Work out the finished part from the listing and answer in its coordinate system (mm). Round coordinates to 2 decimals unless told otherwise and drop trailing zeros. Order: outer loops, then holes, each group sorted by start corner. A loop starts at its lowest first (then second) coordinate and runs counter-clockwise, first axis right, second up. Notation, with made-up numbers: (-28.5, 76.25) - (12.5, 76.25) arc R17 cw to (12.5, 81.25) - close; hole circle Ø8 at (-33, -39.5). An arc over 180 degrees is marked (long way). Put each result on its own line as item: value.
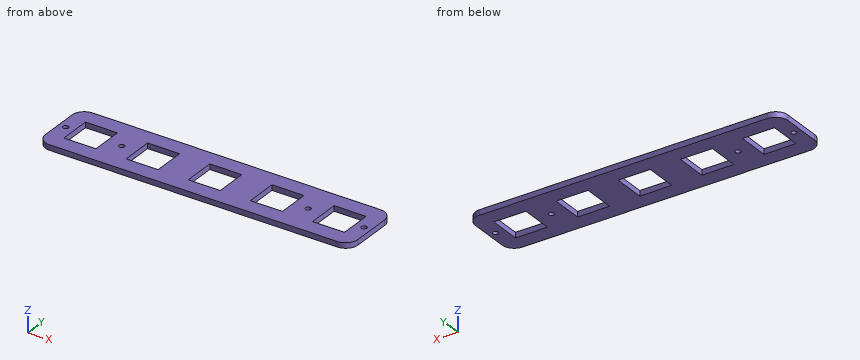
Autodesk Fusion 360 part; units mm, degrees
sketch "Sketch1" plane through (0, 0, 0) normal (0, 0, 1) x (1, 0, 0)
  line L0 (-9, 9) -> (9, 9)
  line L1 (9, 9) -> (9, -9)
  line L2 (9, -9) -> (-9, -9)
  line L3 (-9, -9) -> (-9, 9)
  line L4 (-9, 9) -> (9, -9) construction
  line L5 (9, 9) -> (-9, -9) construction
  line L6 (-81, 18) -> (81, 18)
  line L7 (88, 11) -> (88, -11)
  line L8 (81, -18) -> (-81, -18)
  line L9 (-88, -11) -> (-88, 11)
  line L10 (-88, 18) -> (88, -18) construction
  line L11 (88, 18) -> (-88, -18) construction
  arc A0 (-81, 18) -> (-88, 11) centre (-81, 11) ccw
  arc A1 (-88, -11) -> (-81, -18) centre (-81, -11) ccw
  arc A2 (81, -18) -> (88, -11) centre (81, -11) ccw
  arc A3 (88, 11) -> (81, 18) centre (81, 11) ccw
  line L12 (0, 0) -> (0, 18) construction
  circle A4 centre (-84, 0) radius 1.5
  line L13 (-79, 9) -> (-61, 9)
  line L14 (-79, -9) -> (-79, 9)
  line L15 (-61, -9) -> (-79, -9)
  line L16 (-61, 9) -> (-61, -9)
  line L17 (-44, 9) -> (-26, 9)
  line L18 (-44, -9) -> (-44, 9)
  line L19 (-26, -9) -> (-44, -9)
  line L20 (-26, 9) -> (-26, -9)
  line L21 (26, 9) -> (44, 9)
  line L22 (26, -9) -> (26, 9)
  line L23 (44, -9) -> (26, -9)
  line L24 (44, 9) -> (44, -9)
  line L25 (61, 9) -> (79, 9)
  line L26 (61, -9) -> (61, 9)
  line L27 (79, -9) -> (61, -9)
  line L28 (79, 9) -> (79, -9)
  circle A5 centre (84, 0) radius 1.5
  circle A6 centre (-52.5, 0) radius 1.5
  circle A7 centre (52.5, 0) radius 1.5
  dimension "d22" = 18
  dimension "d23" = 18
  dimension "d28" = 176
  dimension "d29" = 36
  dimension "d30" = 7
  dimension "d35" = 3
  dimension "d36" = 4
  dimension "d37" = 18
  dimension "d44" = 35
  dimension "d45" = 0
  dimension "d60" = 3
  dimension "d61" = 8.5
extrude "Extrude6" add sketch "Sketch1" along normal blind 3
equation "d44 = 17 mm + 18 mm"
equation "d61 = ( 17 / 2 ) * 1 mm"
1) Given pin 1 Ø1.5 at (y, z) = (-12.5, 0.5) entering from +X, flat-ended and moving along its own axis, determine where the tip first touches the part or whether it passes through.
Findings below:
pin 1: stops at x = 87.96
2) Straight lines are drawn through the part: L1, parallel to Y at x = 66.5, z = 0.75; L2, parallel to Y at x = -52.5, z = 2.4; L3, parallel to X at y = -8.5, z = 2. For each, find the intervals that lie inside material, in ascending order. Write a range as from..to.
Findings below:
L1: y = -18..-9, 9..18
L2: y = -18..-1.5, 1.5..18
L3: x = -88..-79, -61..-44, -26..-9, 9..26, 44..61, 79..88
3) A cutting plane is placed at A-A on y = -3. Write down the section's boundary in (x, z).
Findings below:
outline: (-88, 0) - (-79, 0) - (-79, 3) - (-88, 3) - close; (-61, 0) - (-44, 0) - (-44, 3) - (-61, 3) - close; (-26, 0) - (-9, 0) - (-9, 3) - (-26, 3) - close; (9, 0) - (26, 0) - (26, 3) - (9, 3) - close; (44, 0) - (61, 0) - (61, 3) - (44, 3) - close; (79, 0) - (88, 0) - (88, 3) - (79, 3) - close
4) A cutting plane is placed at B-B on x = -52.5. Write down the section's boundary in (y, z).
Findings below:
outline: (-18, 0) - (-1.5, 0) - (-1.5, 3) - (-18, 3) - close; (1.5, 0) - (18, 0) - (18, 3) - (1.5, 3) - close
5) A cutting plane is placed at C-C on z = 1.65. Give the number of separate pieces and of enclosed holes in the cut face, then the cut area to 3 significant figures.
Findings below:
separate pieces: 1
enclosed holes: 9
area: 4,650 mm2
6) A cutting plane is placed at D-D on x = 84. Write down the section's boundary in (y, z), then the cut area to 3 significant figures.
Findings below:
outline: (-17.32, 0) - (-1.5, 0) - (-1.5, 3) - (-17.32, 3) - close; (1.5, 0) - (17.32, 0) - (17.32, 3) - (1.5, 3) - close
area: 94.9 mm2
